from build123d import *

# Parameters (mm, degrees)
F0_W      = 900
F0_H      = 760
F1_DEPTH  = 1400
F2_W      = 900
F2_H      = 640
F3_DEPTH  = 900
F4_W      = 900
F4_H      = 120
F4_H_2    = 30
F5_DEPTH  = 30
F7_DEPTH  = 20
F8_W      = 560
F8_H      = 50
F9_DEPTH  = 50
F10_W     = 250
F10_H     = 170
F11_DEPTH = 600
F12_W     = 560
F12_H     = 420
F13_DEPTH = 600
F14_W     = 400
F14_H     = 100
F15_DEPTH = 300


with BuildPart() as f1:
    # F0 (on Top) → F1 (new body)
    with BuildSketch(Plane.XY):
        with Locations((-172.5741102403, -380)):
            Rectangle(F0_W, F0_H)
    extrude(amount=F1_DEPTH)

    # F2 (on face) → F3 (join)
    with BuildSketch(Plane.XY.offset(1400)):
        with Locations((-172.5741102403, -320)):
            Rectangle(F2_W, F2_H)
    extrude(amount=F3_DEPTH)

    # F4 (on face) → F5 (join)
    with BuildSketch(Plane.XY.offset(1400)):
        with Locations((-172.5741102403, -700)):
            Rectangle(F4_W, F4_H)
        with Locations((-172.5741102403, -775)):
            Rectangle(F4_W, F4_H_2)
    extrude(amount=F5_DEPTH)

    # F6 (on face) → F7 (join)
    with BuildSketch(Plane.XZ.offset(760)):
        Polygon((-452.5741102403, 340), (-452.5741102403, 390), (-452.5741102403, 810), (-452.5741102403, 910), (-502.5741102403, 910), (-502.5741102403, 340), align=None)
        Polygon((107.4258897597, 810), (107.4258897597, 390), (107.4258897597, 340), (157.4258897597, 340), (157.4258897597, 910), (107.4258897597, 910), align=None)
    extrude(amount=F7_DEPTH)

    # F8 (on face) → F9 (join)
    with BuildSketch(Plane.XZ.offset(760)):
        with Locations((-172.5741102403, 365)):
            Rectangle(F8_W, F8_H)
    extrude(amount=F9_DEPTH)

    # F10 (on face) → F11 (cut)
    with BuildSketch(Plane.XZ.offset(760)):
        with Locations((-172.5741102403, 255)):
            Rectangle(F10_W, F10_H)
    extrude(amount=-F11_DEPTH, mode=Mode.SUBTRACT)

    # F12 (on face) → F13 (cut)
    with BuildSketch(Plane.XZ.offset(760)):
        with Locations((-172.5741102403, 600)):
            Rectangle(F12_W, F12_H)
    extrude(amount=-F13_DEPTH, mode=Mode.SUBTRACT)

    # F14 (on face) → F15 (cut)
    with BuildSketch(Plane.XZ.offset(760)):
        with Locations((-172.5741102403, 1350)):
            Rectangle(F14_W, F14_H)
    extrude(amount=-F15_DEPTH, mode=Mode.SUBTRACT)


solid = f1.part
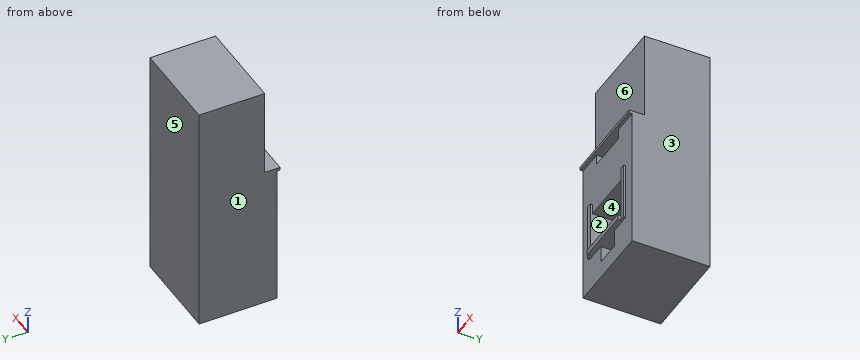
Work out the finished part from the listing and answer in its coordinate system (mm). Face numbers are marked on the shaded views. A direction names the side the tool comes from. Round coordinates to 2 decimals unless told otherwise and drop trailing zeros. Write each loop counter-clockwise with the first axis right and the second up, starting at its lowest first coordinate (ties: lowest second). Pieces come first, ordered by that corner, then holes.
1) A cutting plane is placed at C-C (y = -548). Give the vertices of the cut face in (x, z), plus the area to 3 significant figures.
2) A cutting plane is placed at A-A (y = -279.5). Give the vertices of the cut face in (x, z), plus the area to 3 significant figures.
3) Straight lines are drawn through the part: line 1 (Z direction, x = -254.5, y = -217); line 2 (Z direction, x = -268, y = -580.5); line 3 (Z direction, x = -38.5, y = -674.5). For each, find the intervals that lie inside material, in ascending order.
4) A tool of negligible diameter and unlimited length cuts with its end or side. For the marked faces 5 and 6, from which of +Z, -Z, +X, -X, +Y, -Y can it reach the whole face along a straight path? Write none if from no direction.
5) Given pin 1 Ø1.5 at (x, z) = (136.5, 2028.5) entering from -Y; pin 2 Ø22 at (y, z) = (-772, 602) entering from -X; pin 3 Ø25 at (x, z) = (141, 598) entering from -Y, each flat-ended and moving along its own axis, determine where each tip first touches the part or whether it passes through.
6) A cutting plane is placed at D-D (z = 512.5). Give the vertices of the cut face in (x, y), plus the area to 3 significant figures.
7) A cutting plane is placed at B-B (x = -329). Give the vertices of the cut face in (y, z), plus the area to 4 significant figures.
8) The mould has two halves that part along X. Classify the marked faces 1, 2, 3 and 4: pulls with the +X half, pulls with the -X half, needs draft (parallel to the pull), parting line crosses it, or undercut.
Completed:
1. outline: (-622.57, 0) - (277.43, 0) - (277.43, 2300) - (-622.57, 2300) - close; hole (-452.57, 390) - (107.43, 390) - (107.43, 810) - (-452.57, 810) - close; hole (-372.57, 1300) - (27.43, 1300) - (27.43, 1400) - (-372.57, 1400) - close; hole (-297.57, 170) - (-47.57, 170) - (-47.57, 340) - (-297.57, 340) - close
1. area: 1,750,000 mm2
2. outline: (-622.57, 0) - (277.43, 0) - (277.43, 2300) - (-622.57, 2300) - close; hole (-452.57, 390) - (107.43, 390) - (107.43, 810) - (-452.57, 810) - close; hole (-297.57, 170) - (-47.57, 170) - (-47.57, 340) - (-297.57, 340) - close
2. area: 1,790,000 mm2
3. line 1: z = 0 to 170, 340 to 390, 810 to 2300
3. line 2: z = 0 to 170, 340 to 390, 810 to 1300, 1400 to 2300
3. line 3: z = 0 to 390, 810 to 1300, 1400 to 1430
4. face 5: +Z, -Z, +X, -X, +Y
4. face 6: +Z, +X, -X, -Y
5. pin 1: stops at y = -640
5. pin 2: stops at x = -502.57
5. pin 3: stops at y = -780
6. outline: (-622.57, -760) - (-502.57, -760) - (-502.57, -780) - (-452.57, -780) - (-452.57, -160) - (107.43, -160) - (107.43, -780) - (157.43, -780) - (157.43, -760) - (277.43, -760) - (277.43, 0) - (-622.57, 0) - close
6. area: 350,000 mm2
7. outline: (-810, 340) - (-760, 340) - (-760, 0) - (0, 0) - (0, 2300) - (-640, 2300) - (-640, 1430) - (-790, 1430) - (-790, 1400) - (-460, 1400) - (-460, 1300) - (-760, 1300) - (-760, 810) - (-160, 810) - (-160, 390) - (-810, 390) - close
7. area: 1,365,000 mm2
8. face 1: pulls with the -X half
8. face 2: undercut
8. face 3: pulls with the +X half
8. face 4: undercut
